Here's how the part is built. I have some questions about the finished solid (model axes, mm). Give positions to 0.01 mm unless a question says otherwise; leave off trailing zeros. Write each loop counter-clockwise with the first axis right and the second up, starting at its lowest first coordinate (ties: lowest second). Pieces come first, ordered by that corner, then holes. Notation, with made-up numbers: (-15.75, 57.5) -> (27.25, 57.5) arc R17 ccw to (27.25, 85.5) -> close; hole circle Ø2 at (85.5, 79.25). An arc over 180 degrees is marked (long way). Use CSV: the item, a comma, the result in double quotes. Start each with the question number.
(1) Suppose I cut it at C-C on y = -25. List the corners of the cut face in (x, z) for me.
(2) Suppose I cut it at A-A on z = 4. List the corners of the cut face in (x, y) for me.
(3) Suppose I cut it at D-D on x = -107. List the corners of the cut face in (y, z) for me, plus the area to 3 significant figures.
(4) Suppose I cut it at B-B on x = 43. List the corners of the cut face in (y, z) for me.
(5) For pin 1 Ø2 at (y, z) = (21, 5.5) entering from +X; pin 2 Ø2 at (x, z) = (-34, 2.5) entering from +Y; pin 3 Ø3 at (x, z) = (-62.5, 3) entering from -Y, each with a flat end and sliding along its axis, tell me the tip position at first contact or that it passes through.
(6) I need wall thicknesses on L1, parallel to X at y = 4.5, z = 6; L2, parallel to X at y = 0, z = 5.75; L3, parallel to X at y = 29.5, z = 4. Which ranges of each line are inside material? Lowest first, please. Write a range as [from, to].
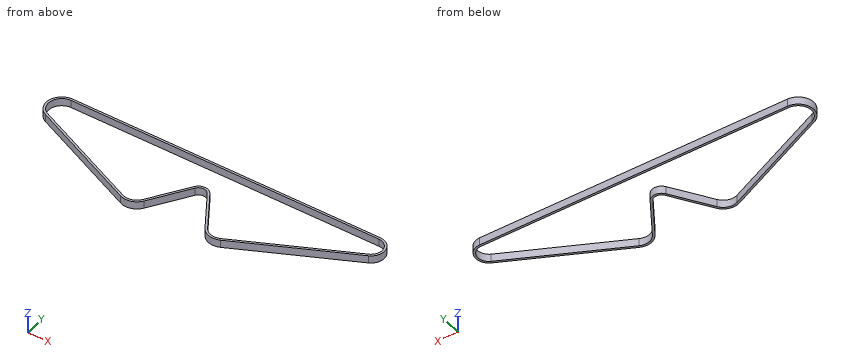
from build123d import *

# Parameters (mm, degrees)
BOSS_EXTRUDE1_DEPTH = 7


with BuildPart() as part:
    # Sketch4 → Boss-Extrude1 (new body)
    with BuildSketch(Plane.XY):
        with BuildLine():
            Line((149.215463732, 12.793345832), (46.589393766, -36.607849916))
            ThreePointArc((46.589393766, -36.607849916), (36.535868579, -37.486862399), (28.414970428, -31.495448136))
            Line((28.414970428, -31.495448136), (5.685960057, 3.674609943))
            ThreePointArc((5.685960057, 3.674609943), (0, 6.77), (-5.685960057, 3.674609943))
            Line((-5.685960057, 3.674609943), (-28.414970428, -31.495448136))
            ThreePointArc((-28.414970428, -31.495448136), (-36.408809792, -37.450485427), (-46.350175166, -36.720285855))
            Line((-46.350175166, -36.720285855), (-149.891425293, 10.779714145))
            ThreePointArc((-149.891425293, 10.779714145), (-157.871281998, 26.846306071), (-143.836659858, 38.019616704))
            Line((-143.836659858, 38.019616704), (144.030375349, 35.909673379))
            ThreePointArc((144.030375349, 35.909673379), (155.806430283, 26.411409249), (149.215463732, 12.793345832))
        make_face()
        with BuildLine():
            Line((-143.851318616, 36.019670425), (144.015716591, 33.9097271))
            ThreePointArc((144.015716591, 33.9097271), (153.854920385, 25.973677464), (148.347994384, 14.59542711))
            Line((148.347994384, 14.59542711), (45.721924419, -34.805768638))
            ThreePointArc((45.721924419, -34.805768638), (37.077442705, -35.561583857), (30.094722291, -30.409891285))
            Line((30.094722291, -30.409891285), (7.36571192, 4.760166794))
            ThreePointArc((7.36571192, 4.760166794), (0, 8.77), (-7.36571192, 4.760166794))
            Line((-7.36571192, 4.760166794), (-30.094722291, -30.409891285))
            ThreePointArc((-30.094722291, -30.409891285), (-36.968191738, -35.530305269), (-45.516233303, -34.902446212))
            Line((-45.516233303, -34.902446212), (-149.05748343, 12.597553788))
            ThreePointArc((-149.05748343, 12.597553788), (-155.918929945, 26.412345864), (-143.851318616, 36.019670425))
        make_face(mode=Mode.SUBTRACT)
    extrude(amount=BOSS_EXTRUDE1_DEPTH)


solid = part.part
Geometry says:
1,outline,"(-71.9, 0) -> (-67.1, 0) -> (-67.1, 7) -> (-71.9, 7) -> close; (-26.6, 0) -> (-24.22, 0) -> (-24.22, 7) -> (-26.6, 7) -> close; (24.22, 0) -> (26.6, 0) -> (26.6, 7) -> (24.22, 7) -> close; (66.09, 0) -> (70.7, 0) -> (70.7, 7) -> (66.09, 7) -> close"
2,outline,"(-149.89, 10.78) -> (-46.35, -36.72) arc R14.27 ccw to (-28.41, -31.5) -> (-5.69, 3.67) arc R6.77 cw to (5.69, 3.67) -> (28.41, -31.5) arc R14.27 ccw to (46.59, -36.61) -> (149.22, 12.79) arc R12.16 ccw to (144.03, 35.91) -> (-143.84, 38.02) arc R14.27 ccw to start; hole (-149.06, 12.6) -> (-45.52, -34.9) arc R12.27 ccw to (-30.09, -30.41) -> (-7.37, 4.76) arc R8.77 cw to (7.37, 4.76) -> (30.09, -30.41) arc R12.27 ccw to (45.72, -34.81) -> (148.35, 14.6) arc R10.16 ccw to (144.02, 33.91) -> (-143.85, 36.02) arc R12.27 ccw to start"
3,outline,"(-8.9, 0) -> (-6.7, 0) -> (-6.7, 7) -> (-8.9, 7) -> close; (35.75, 0) -> (37.75, 0) -> (37.75, 7) -> (35.75, 7) -> close"
3,area,"29.4 mm²"
4,outline,"(-37.78, 0) -> (-35.74, 0) -> (-35.74, 7) -> (-37.78, 7) -> close; (34.65, 0) -> (36.65, 0) -> (36.65, 7) -> (34.65, 7) -> close"
5,pin 1,"x = 155.97"
5,pin 2,"y = 37.22"
5,pin 3,"y = -30"
6,L1,"[-136.2, -131.41], [-7.53, -5.06], [5.06, 7.53], [127.38, 131.99]"
6,L2,"[-126.39, -121.6], [-10.44, -8.06], [8.06, 10.44], [118.03, 122.64]"
6,L3,"[-157, -154.78], [152.32, 154.66]"
